```python
from build123d import *

# Parameters (mm, degrees)
SKETCH2_OUTSIDE_W  = 27.658
SKETCH2_OUTSIDE_H  = 27.658
CUT_EXTRUDE1_DEPTH = 7.9
FILLET1_R          = 0.5
FILLET2_R          = 0.8


with BuildPart() as part:
    # Sketch1 → Revolve1 (revolve)
    with BuildSketch(Plane.XY, mode=Mode.PRIVATE) as revolve1_sk:
        Polygon((0, 5.25), (0, 7), (-0.401923789, 8.5), (-7.9, 8.5), (-7.9, 9.75), (-13.7, 9.75), (-13.7, 5.25), (-12.7, 4.25), (-1, 4.25), align=None)
    revolve(revolve1_sk.sketch.rotate(Axis((0, 0, 0), (-1, 0, 0)), 90), axis=Axis((0, 0, 0), (-1, 0, 0)))

    # Sketch2 outside → Cut-Extrude1 (cut)
    with BuildSketch(Plane(origin=(0, 0, 0), x_dir=(0, 0, -1), z_dir=(1, 0, 0))):
        Rectangle(SKETCH2_OUTSIDE_W, SKETCH2_OUTSIDE_H)
        Polygon((8.660254038, 0), (4.330127019, 7.5), (-4.330127019, 7.5), (-8.660254038, 0), (-4.330127019, -7.5), (4.330127019, -7.5), align=None, mode=Mode.SUBTRACT)
    extrude(amount=-CUT_EXTRUDE1_DEPTH, mode=Mode.SUBTRACT)

    # Fillet1
    fillet1_edges = [part.edges().sort_by_distance(p)[0] for p in [
        (-7.9, 0, 9.75),
        (-13.7, 0, 9.75),
    ]]
    fillet(fillet1_edges, radius=FILLET1_R)

    # Fillet2
    fillet2_edges = [part.edges().sort_by_distance(p)[0] for p in [
        (-7.9, 3.75, -6.495190528),
        (-7.9, 7.5, 0),
        (-7.9, 3.75, 6.495190528),
        (-7.9, -3.75, 6.495190528),
        (-7.9, -7.5, 0),
        (-7.9, -3.75, -6.495190528),
    ]]
    fillet(fillet2_edges, radius=FILLET2_R)


solid = part.part
```
The listing builds one solid part. Answer for the finished solid, in the listing's coordinates (mm). A direction names the side the tool comes from. Give positions to 0.01 mm unless a question says otherwise; leave off trailing zeros. Order: outer loops, then holes, each group sorted by start corner. A loop starts at its lowest first (then second) coordinate and runs counter-clockwise, first axis right, second up. Notation, with made-up numbers: (-26.75, -2.5) -> (-0.75, -2.5) arc R4 ccw to (-0.75, 4.5) -> close; hole circle Ø8 at (61.25, 30.5). An arc over 180 degrees is marked (long way). Write each question's results on one line, items separated by ' | '.
Q1. Each of these flat-tipped pins is pushed along its axis until it touches: P1, Ø2, axis at x = -5, z = 2, coming from the -Y side; P2, Ø5.5, axis at x = -4.5, z = -1, coming from the +Y side; P3, Ø4, axis at x = -11, y = 2.5, coming from the +Z side. Where does it stop, or does it pass through?
Checked values:
P1: stops at y = -7.5 | P2: stops at y = 7.51 | P3: stops at z = 9.74
Q2. Straight lines are drawn through the part: probe 1 along Y at (x, z) = (-5.5, 0); probe 2 along Y at (x, z) = (-8.75, 0); probe 3 along Z at (x, y) = (-6.75, 1.25). For each, find the intervals that lie inside material, in ascending order. Write a range as from..to.
Checked values:
probe 1: y = -7.5..-4.25, 4.25..7.5 | probe 2: y = -9.75..-4.25, 4.25..9.75 | probe 3: z = -7.94..-4.06, 4.06..7.94
Q3. The part is cut by section A-A, the plane y = 0. Give the vertices of the cut face in (x, z).
Checked values:
outline: (-13.7, -9.25) arc R0.5 ccw to (-13.2, -9.75) -> (-8.4, -9.75) arc R0.5 ccw to (-7.9, -9.25) -> (-7.9, -8.5) -> (-0.4, -8.5) -> (0, -7) -> (0, -5.25) -> (-1, -4.25) -> (-12.7, -4.25) -> (-13.7, -5.25) -> close; (-13.7, 5.25) -> (-12.7, 4.25) -> (-1, 4.25) -> (0, 5.25) -> (0, 7) -> (-0.4, 8.5) -> (-7.9, 8.5) -> (-7.9, 9.25) arc R0.5 ccw to (-8.4, 9.75) -> (-13.2, 9.75) arc R0.5 ccw to (-13.7, 9.25) -> close
Q4. The part is cut by section D-D, the plane x = -12.25. Give the vertices of the cut face in (y, z), and give its area (3 significant figures).
Checked values:
outline: circle Ø19.5 at (0, 0); hole circle Ø8.5 at (0, 0) | area: 242 mm^2
Q5. The part is cut by section C-C, the plane z = 0. Give the vertices of the cut face in (x, y), and give its area (3 significant figures).
Checked values:
outline: (-13.7, -9.25) arc R0.5 ccw to (-13.2, -9.75) -> (-8.4, -9.75) arc R0.5 ccw to (-7.9, -9.25) -> (-7.9, -8.3) arc R0.8 cw to (-7.1, -7.5) -> (-0.13, -7.5) -> (0, -7) -> (0, -5.25) -> (-1, -4.25) -> (-12.7, -4.25) -> (-13.7, -5.25) -> close; (-13.7, 5.25) -> (-12.7, 4.25) -> (-1, 4.25) -> (0, 5.25) -> (0, 7) -> (-0.13, 7.5) -> (-7.1, 7.5) arc R0.8 cw to (-7.9, 8.3) -> (-7.9, 9.25) arc R0.5 ccw to (-8.4, 9.75) -> (-13.2, 9.75) arc R0.5 ccw to (-13.7, 9.25) -> close | area: 113 mm^2
Q6. The part is cut by section B-B, the plane x = -6.75. Give the vertices of the cut face in (y, z), and give its area (3 significant figures).
Checked values:
outline: (-7.5, -4) arc R8.5 ccw to (-7.21, -4.5) -> (-0.29, -8.5) arc R8.5 ccw to (0.29, -8.5) -> (7.21, -4.5) arc R8.5 ccw to (7.5, -4) -> (7.5, 4) arc R8.5 ccw to (7.21, 4.5) -> (0.29, 8.5) arc R8.5 ccw to (-0.29, 8.5) -> (-7.21, 4.5) arc R8.5 ccw to (-7.5, 4) -> close; hole circle Ø8.5 at (0, 0) | area: 138 mm^2
Q7. Which of the six approach directions +Z, -Z, +X, -X, +Y, -Y give full straight-line access (tool end or side, diameter ignored) to faces 1 (the face through (-3.568, -3.798, -6.467)), 2 (the face through (-4.724, 7.367, -4.239)), 3 (the face through (-4.724, -7.367, 4.239)), 4 (the face through (-4, -7.5, 0))?
Checked values:
face 1: -Z, +X, -Y | face 2: -Z, +X, +Y | face 3: +Z, +X, -Y | face 4: +Z, -Z, +X, -Y
